from build123d import *

# Parameters (mm, degrees)
SKETCH1_W                             = 381
SKETCH1_H                             = 25.4
BOSS_EXTRUDE1_DEPTH                   = 3.175
F_1_4_CLEARANCE_FIRST_MOUNTING_HOLE_D = 6.7564
PEDAL_BOX_MOUNTING_HOLE_PATTERN_COUNT = 15
PEDAL_BOX_MOUNTING_HOLE_PATTERN_PITCH = 25.4
SKETCH8_W                             = 3.175
SKETCH8_H                             = 12.7
SUPPORT_TAB_WELDING_CUT_DEPTH         = 3.175
SUPPORT_TAB_WELDING_CUT_PATTERN_COUNT = 4
SUPPORT_TAB_WELDING_CUT_PATTERN_PITCH = 76.2


with BuildPart() as part:
    # Sketch1 → Boss-Extrude1 (new body)
    with BuildSketch(Plane(origin=(0, 0, 0), x_dir=(1, 0, 0), z_dir=(0, 1, 0))):
        with Locations((190.5, 12.7)):
            Rectangle(SKETCH1_W, SKETCH1_H)
    extrude(amount=BOSS_EXTRUDE1_DEPTH)

    # 1/4 Clearance First Mounting Hole (through all)
    with Locations(Plane(origin=(0, 3.175, 0), x_dir=(1, 0, 0), z_dir=(0, 1, 0))):
        with Locations((12.7, 12.7)):
            f_1_4_clearance_first_mounting_hole = Hole(F_1_4_CLEARANCE_FIRST_MOUNTING_HOLE_D / 2)

    # Pedal Box Mounting Hole Pattern: 1/4 Clearance First Mounting Hole ×15
    with Locations(*[(i * PEDAL_BOX_MOUNTING_HOLE_PATTERN_PITCH, 0, 0) for i in range(1, PEDAL_BOX_MOUNTING_HOLE_PATTERN_COUNT)]):
        add(f_1_4_clearance_first_mounting_hole, mode=Mode.SUBTRACT)

    # Sketch8 → Support Tab Welding Cut (cut)
    with BuildSketch(Plane(origin=(0, 3.175, 0), x_dir=(1, 0, 0), z_dir=(0, 1, 0))):
        with Locations((76.2, 12.7)):
            Rectangle(SKETCH8_W, SKETCH8_H)
    support_tab_welding_cut = extrude(amount=-SUPPORT_TAB_WELDING_CUT_DEPTH, mode=Mode.SUBTRACT)

    # Support Tab Welding Cut Pattern: Support Tab Welding Cut ×4
    with Locations(*[(i * SUPPORT_TAB_WELDING_CUT_PATTERN_PITCH, 0, 0) for i in range(1, SUPPORT_TAB_WELDING_CUT_PATTERN_COUNT)]):
        add(support_tab_welding_cut, mode=Mode.SUBTRACT)


solid = part.part
Geometry check sheet. Reference: the model listing, model coordinates, mm. Round coordinates to 2 decimals unless told otherwise and drop trailing zeros. Loops run counter-clockwise (first coordinate to the right, second up) from the corner with the lowest first, then second, coordinate; pieces in that order, holes last.
Item 1: Mould release check, pull along X, two halves, no side actions. Record for faces 1 (the cylindrical face through (371.675, 1.565, -12.849)), 2 (the flat face through (188, 3.175, -10)), 3 (the cylindrical face through (64.23, 1.57, -9.4)): pulls with the +X half, pulls with the -X half, needs draft (parallel to the pull), parting line crosses it, or undercut.
Item 2: Thickness scan on line 1 (X direction, y = 0.3, z = -8.5); line 2 (Z direction, x = 241.3, y = 1.7); line 3 (Z direction, x = 153, y = 1.15). Record the ranges inside material, lowest first.
Item 3: Cross-section at B-B on z = -12.7. Count the separate pieces of the cut face and the enclosed holes in it, then the cut area to 3 significant figures.
Item 4: Cross-section at A-A on x = 241.3. Record the boundary of the cut face in (y, z) (3 decimals).
Answer sheet:
1. face 1: undercut
1. face 2: needs draft
1. face 3: undercut
2. line 1: x = 0 to 74.61, 77.79 to 150.81, 153.99 to 227.01, 230.19 to 303.21, 306.39 to 381
2. line 2: z = -25.4 to -16.08, -9.32 to 0
2. line 3: z = -25.4 to -19.05, -6.35 to 0
3. separate pieces: 20
3. enclosed holes: 0
3. area: 848 mm2
4. outline: (0, -25.4) - (3.175, -25.4) - (3.175, -16.078) - (0, -16.078) - close; (0, -9.322) - (3.175, -9.322) - (3.175, 0) - (0, 0) - close
